```python
from build123d import *

# Parameters (mm, degrees)
F0_W     = 115
F0_H     = 15
F1_DEPTH = 5
F2_R     = 7.5
F3_DEPTH = 15


with BuildPart() as f1:
    # F0 (on Top) → F1 (new body)
    with BuildSketch(Plane.XY):
        Rectangle(F0_W, F0_H)
    extrude(amount=F1_DEPTH)

    # F2 (on face) → F3 (join)
    with BuildSketch(Plane.XY.offset(5)):
        with BuildLine():
            ThreePointArc((-57.5, 0), (-50, -7.5), (-42.5, 0))
            ThreePointArc((-42.5, 0), (-50, 7.5), (-57.5, 0))
        make_face()
        with Locations((50, 0)):
            Circle(F2_R)
    extrude(amount=F3_DEPTH)


solid = f1.part
```
Source: CAD feature listing. Evaluate the final solid. Frame: model axes, mm. A direction names the side the tool comes from. Give positions to 0.01 mm unless a question says otherwise; leave off trailing zeros. Loops run counter-clockwise (first coordinate to the right, second up) from the corner with the lowest first, then second, coordinate; pieces in that order, holes last. Notation, with made-up numbers: (-36.5, 50.5) -> (-18.5, 50.5) arc R14 ccw to (-18.5, 68.5) -> close; hole circle Ø7 at (62.25, 29). An arc over 180 degrees is marked (long way). Put each result on its own line as item: value. Start each with the question number.
1) Draft query along X for faces 1 (the face through (57.154, 2.253, 12.395)), 2 (the face through (56, -6, 5)), 3 (the face through (57.5, 0, 2)). Return one class per face: released by +X, released by -X, zero draft, split by the parting line, or undercut.
2) Reachability of faces 4 (the face through (-56, -6, 5)), 5 (the face through (-56, 6, 5)), 6 (the face through (56, 6, 5)), 7 (the face through (50, 0, 20)), 8 (the face through (-42.846, 2.253, 12.395)) from +Z, -Z, +X, -X, +Y, -Y: full face, straight path, thin tool, end or side. Return the list, or none.
3) Cut plane D-D (y = -3.5). Return loops of the section in (x, z).
4) Cut plane A-A (y = 6). Return loops of the section in (x, z), then the cut area to 3 significant figures.
5) Cut plane C-C (x = 5). Return loops of the section in (y, z), then the cut area to 3 significant figures.
6) Material intervals for probe 1 along Z at (x, y) = (-32.5, 2); probe 2 along X at (y, z) = (6.5, 16); probe 3 along Y at (x, z) = (-50.5, 15.5), sorted ascending.
7) Cut plane B-B (z = 6.5). Return loops of the section in (x, y).
8) Contact query for flat-ended pins moving along their axis: P1, Ø6, axis at x = 30, y = -1.5, coming from the +Z side; P2, Ø2, axis at y = 1.5, z = 17, coming from the +X side; P3, Ø3, axis at y = -1, z = 13, coming from the -X side; P4, Ø1, axis at x = 31, z = 6.5, coming from the -Y side. Output: stop coordinate, or through.
Results are:
1. face 1: undercut
1. face 2: zero draft
1. face 3: released by +X
2. face 4: +Z, -X, -Y
2. face 5: +Z, -X, +Y
2. face 6: +Z, +X, +Y
2. face 7: +Z, +X, -X, +Y, -Y
2. face 8: +Z
3. outline: (-57.5, 0) -> (57.5, 0) -> (57.5, 5) -> (56.63, 5) -> (56.63, 20) -> (43.37, 20) -> (43.37, 5) -> (-43.37, 5) -> (-43.37, 20) -> (-56.63, 20) -> (-56.63, 5) -> (-57.5, 5) -> close
4. outline: (-57.5, 0) -> (57.5, 0) -> (57.5, 5) -> (54.5, 5) -> (54.5, 20) -> (45.5, 20) -> (45.5, 5) -> (-45.5, 5) -> (-45.5, 20) -> (-54.5, 20) -> (-54.5, 5) -> (-57.5, 5) -> close
4. area: 845 mm2
5. outline: (-7.5, 0) -> (7.5, 0) -> (7.5, 5) -> (-7.5, 5) -> close
5. area: 75.0 mm2
6. probe 1: z = 0 to 5
6. probe 2: x = -53.74 to -46.26, 46.26 to 53.74
6. probe 3: y = -7.48 to 7.48
7. outline: circle Ø15 at (-50, 0); circle Ø15 at (50, 0)
8. P1: stops at z = 5
8. P2: stops at x = 57.48
8. P3: stops at x = -57.5
8. P4: passes through
